Verification items for the finished model (mm, model axes). A direction names the side the tool comes from. Give positions to 0.01 mm unless a question says otherwise; leave off trailing zeros. Order: outer loops, then holes, each group sorted by start corner. A loop starts at its lowest first (then second) coordinate and runs counter-clockwise, first axis right, second up. Notation, with made-up numbers: (-6, 4) - (38, 4) arc R29 ccw to (38, 39) - close; hole circle Ø3 at (-0.75, 28). An arc over 180 degrees is marked (long way). Answer as a JSON object with one key per item and string values. Group by question number.
(1) Section check B-B (x = -42.5). Record the boundary of the cut face in (y, z), then the cut area to 3 significant figures.
(2) Section check C-C (x = -13). Record the boundary of the cut face in (y, z).
(3) Thickness scan on line 1 (X direction, y = 5.25, z = 0); line 2 (X direction, y = 1.7, z = 0); line 3 (Z direction, x = -41.5, y = 1.25). Record the ranges inside material, lowest first.
(4) Section check A-A (z = 0). Count the separate pieces of the cut face and the enclosed holes in it, then the cut area to 3 significant figures.
(5) Mould release check, pull along X, two halves, no side actions. Record for faces 1 (the face through (-60.7, 7.8, 0.4)), 2 (the face through (46.726, 6.712, -0.923)), 3 (the face through (-23, 8, -23)): +X half, -X half, draft (parallel to the pull), parting line (faces both ways), or undercut.
(6) Section check D-D (x = 48.5). Record the boundary of the cut face in (y, z).
(7) Access from +Z, -Z, +X, -X, +Y, -Y to the whole of each face (thin tool, end or side, straight path). Record for faces 4 (the face through (-1, 8, 23)), 5 (the face through (-44, 4, -2)), 6 (the face through (34.8, 2.5, -19.1)).
(8) Depth check by flat-ended pin: pin 1 Ø4.5 at (x, z) = (48.5, 0) entering from +Y; pin 2 Ø2.5 at (x, z) = (-41.5, 1) entering from -Y; pin 3 Ø3 at (x, y) = (-19.5, 8) entering from -Z. Enter the tip coordinate at first touch or a pass-through.
```python
from build123d import *

# Parameters (mm, degrees)
SKETCH1_W           = 125
SKETCH1_H           = 50
BOSS_EXTRUDE1_DEPTH = 9.5
CHAMFER1_SIZE       = 3.5
SKETCH3_R           = 4
CUT_EXTRUDE2_DEPTH  = 4
SKETCH4_R           = 2
CUT_EXTRUDE3_DEPTH  = 68.538877693
SKETCH6_R           = 43
CUT_EXTRUDE4_DEPTH  = 12


with BuildPart() as part:
    # Sketch1 → Boss-Extrude1 (new body)
    with BuildSketch(Plane(origin=(0, 0, 0), x_dir=(1, 0, 0), z_dir=(0, 1, 0))):
        Rectangle(SKETCH1_W, SKETCH1_H)
    extrude(amount=BOSS_EXTRUDE1_DEPTH)

    # Chamfer1
    chamfer1_edges = [part.edges().sort_by_distance(p)[0] for p in [
        (-62.5, 9.5, 0),
        (0, 9.5, 25),
        (62.5, 9.5, 0),
        (0, 9.5, -25),
    ]]
    chamfer(chamfer1_edges, length=CHAMFER1_SIZE)

    # Sketch3 → Cut-Extrude2 (cut)
    with BuildSketch(Plane.XZ):
        with Locations(Location((-42.5, 0, 0), (0, 0, 270))):
            Circle(SKETCH3_R)
        with Locations(Location((20.5, 0, 0), (0, 0, 270))):
            Circle(SKETCH3_R)
        with Locations(Location((48.5, 0, 0), (0, 0, 270))):
            Circle(SKETCH3_R)
    extrude(amount=-CUT_EXTRUDE2_DEPTH, mode=Mode.SUBTRACT)

    # Sketch4 → Cut-Extrude3 (cut, through all)
    with BuildSketch(Plane.XZ.offset(-4)):
        with Locations(Location((-42.5, 0, 0), (0, 0, 270))):
            Circle(SKETCH4_R)
        with Locations(Location((20.5, 0, 0), (0, 0, 270))):
            Circle(SKETCH4_R)
        with Locations(Location((48.5, 0, 0), (0, 0, 270))):
            Circle(SKETCH4_R)
    extrude(amount=-CUT_EXTRUDE3_DEPTH, mode=Mode.SUBTRACT)

    # Sketch6 → Cut-Extrude4 (cut)
    with BuildSketch(Plane(origin=(0, 0, -25), x_dir=(-1, 0, 0), z_dir=(0, 0, -1))):
        with Locations((-34.5, 45.5)):
            Circle(SKETCH6_R)
    extrude(amount=-CUT_EXTRUDE4_DEPTH, mode=Mode.SUBTRACT)


solid = part.part
```
Solutions:
{
 "1": {"outline": "(0, -25) - (6, -25) - (9.5, -21.5) - (9.5, -2) - (4, -2) - (4, -4) - (0, -4) - close; (0, 4) - (4, 4) - (4, 2) - (9.5, 2) - (9.5, 21.5) - (6, 25) - (0, 25) - close", "area": "409 mm2"},
 "2": {"outline": "(0, -25) - (6, -25) - (9.5, -21.5) - (9.5, 21.5) - (6, 25) - (0, 25) - close"},
 "3": {"line 1": "x = -62.5 to -44.5, -40.5 to 18.5, 22.5 to 46.5, 50.5 to 62.5", "line 2": "x = -62.5 to -46.5, -38.5 to 16.5, 24.5 to 44.5, 52.5 to 62.5", "line 3": "z = -25 to -3.87, 3.87 to 25"},
 "4": {"separate pieces": "4", "enclosed holes": "0", "area": "1,010 mm2"},
 "5": {"face 1": "-X half", "face 2": "undercut", "face 3": "draft"},
 "6": {"outline": "(0, -25) - (4.84, -25) - (4.84, -13) - (9.5, -13) - (9.5, -2) - (4, -2) - (4, -4) - (0, -4) - close; (0, 4) - (4, 4) - (4, 2) - (9.5, 2) - (9.5, 21.5) - (6, 25) - (0, 25) - close"},
 "7": {"face 4": "+Z, +X, -X, +Y", "face 5": "-Y", "face 6": "-Z, +Y"},
 "8": {"pin 1": "stops at y = 9.5", "pin 2": "stops at y = 4", "pin 3": "stops at z = -24.5"}
}
